Model file for the job. Use its own axes, mm. A direction names the side the tool comes from. Round coordinates to 2 decimals unless told otherwise and drop trailing zeros. Loops run counter-clockwise (first coordinate to the right, second up) from the corner with the lowest first, then second, coordinate; pieces in that order, holes last. Notation, with made-up numbers: (60.5, 75.25) - (84.5, 75.25) arc R14 cw to (84.5, 97.25) - close; hole circle Ø2 at (58, 79.25). An arc over 180 degrees is marked (long way). Answer as a JSON object with one key per item and string values.
Autodesk Inventor part; units mm, degrees
ref_plane "YZ Plane" through (0, 0, 0) normal (1, 0, 0) x (0, 1, 0)
ref_plane "XZ Plane" through (0, 0, 0) normal (0, 1, 0) x (-1, 0, 0)
ref_plane "XY Plane" through (0, 0, 0) normal (0, 0, 1) x (1, 0, 0)
sketch "Sketch1" plane through (0, 0, 0) normal (0, 1, 0) x (-1, 0, 0)
  line L0 (13.5, 27.25) -> (-13.5, 27.25)
  line L1 (-13.5, 27.25) -> (-13.5, -27.25)
  line L2 (-13.5, -27.25) -> (13.5, -27.25)
  line L3 (13.5, -27.25) -> (13.5, 27.25)
  line L4 (13.5, 27.25) -> (-13.5, -27.25) construction
  line L5 (-13.5, 27.25) -> (13.5, -27.25) construction
  circle A0 centre (16.75, 0) radius 1.5
  circle A1 centre (16.75, 0) radius 4
  line L6 (20.75, -4) -> (12.75, -4)
  line L7 (12.75, -4) -> (12.75, 4)
  line L8 (12.75, 4) -> (20.75, 4)
  line L9 (20.75, 4) -> (20.75, -4)
  line L10 (20.75, -4) -> (12.75, 4) construction
  line L11 (12.75, -4) -> (20.75, 4) construction
  point P0 (0, 0)
  point P1 (16.75, -4)
  point P2 (16.75, 4)
  point P3 (13.5, 4)
  point P4 (13.5, -4)
  dimension "d0" = 54.5
  dimension "d1" = 27
  dimension "d3" = 3
  dimension "d4" = 8
  dimension "d7" = 3.25
extrude "Extrusion1" add sketch "Sketch1" along normal blind 4.5 contours L3 L8 L7 L6 L2 L1 L0 | L8 A1 L3 | L3 A1 L7 L8 | A1 L3 | L3 A1 | A1 L6 L3 | L3 L6 L7 A1
properties part number "Ortak_bat_lid"
1) Two-plate mould, pull along X, no slides. Class faces 1 (the cylindrical face through (-15.25, 2.22, -0.07)), 2 (the cylindrical face through (-20.75, 2.22, 0.09)), 3 (the flat face through (0, 2, -27.25)): pulls with the +X half, pulls with the -X half, needs draft (parallel to the pull), parting line crosses it, or undercut.
Values follow:
{"face 1": "undercut", "face 2": "pulls with the -X half", "face 3": "needs draft"}
2) Slice it at D-D on z = 12. List the corners of the cut face in (x, y), then the cut area to 4 significant figures.
Values follow:
{"outline": "(-13.5, 0) - (13.5, 0) - (13.5, 4.5) - (-13.5, 4.5) - close", "area": "121.5 mm²"}
3) Tool access for faces 4 (the flat face through (-13.5, 2, -16)), 5 (the flat face through (0, 4.5, 0)), 6 (the flat face through (-15, 2, 4)): list every direction of +Z, -Z, +X, -X, +Y, -Y with a clear straight run to the whole face (end or side of a thin tool).
Values follow:
{"face 4": "-Z, -X, +Y, -Y", "face 5": "+Z, -Z, +X, -X, +Y", "face 6": "+Z, -X, +Y, -Y"}
4) Slice it at A-A on z = 0. List the corners of the cut face in (x, y).
Values follow:
{"outline": "(-20.75, 0) - (-18.25, 0) - (-18.25, 4.5) - (-20.75, 4.5) - close; (-15.25, 0) - (13.5, 0) - (13.5, 4.5) - (-15.25, 4.5) - close"}
5) Drop flat-ended pins along their axis: P1, Ø3, axis at x = -15.5, z = -14.5, coming from the -Y side; P2, Ø2.5, axis at x = -15, y = 2.5, coming from the -Z side; P3, Ø2, axis at y = 2, z = -17.5, coming from the -X side; P4, Ø2.5, axis at x = -15.5, y = 3, coming from the +Z side. Give the stop position or say it passes through.
Values follow:
{"P1": "through", "P2": "z = -4", "P3": "x = -13.5", "P4": "z = 4"}
6) Slice it at C-C on x = -16. List the corners of the cut face in (y, z).
Values follow:
{"outline": "(0, -4) - (4.5, -4) - (4.5, -1.3) - (0, -1.3) - close; (0, 1.3) - (4.5, 1.3) - (4.5, 4) - (0, 4) - close"}
7) Slice it at B-B on y = 1.4. List the corners of the cut face in (x, z), then the cut area to 3 significant figures.
Values follow:
{"outline": "(-16.75, -4) - (-13.5, -4) - (-13.5, -27.25) - (13.5, -27.25) - (13.5, 27.25) - (-13.5, 27.25) - (-13.5, 4) - (-16.75, 4) arc R4 ccw to start; hole circle Ø3 at (-16.75, 0)", "area": "1,520 mm²"}
8) Probe probe 1 along Z at (x, y) = (-16.75, 2.15); probe 2 along Z at (x, y) = (-15, 3); probe 3 along X at (y, z) = (1.45, 23.5). List the from-to ranges inside material, lowest first.
Values follow:
{"probe 1": "-4 to -1.5, 1.5 to 4", "probe 2": "-4 to 4", "probe 3": "-13.5 to 13.5"}
